```python
from build123d import *

# Parameters (mm, degrees)
BOSS_EXTRUDE1_DEPTH = 222.57
CUT_EXTRUDE2_START  = -10
CUT_EXTRUDE2_DEPTH  = 10
CUT_EXTRUDE3_START  = -10
CUT_EXTRUDE3_DEPTH  = 10


with BuildPart() as part:
    # Sketch1 → Boss-Extrude1 (new body)
    with BuildSketch(Plane.XY):
        with BuildLine():
            Line((0, 150), (0, 130))
            ThreePointArc((0, 130), (-130, 0), (0, -130))
            Line((0, -130), (0, -150))
            ThreePointArc((0, -150), (-150, 0), (0, 150))
        make_face()
    extrude(amount=BOSS_EXTRUDE1_DEPTH)

    # Sketch2 → Cut-Extrude2 (cut)
    with BuildSketch(Plane.XY.offset(222.57).offset(CUT_EXTRUDE2_START)):
        with BuildLine():
            Line((-10, 129.614813968), (-52.842182765, 129.614813968))
            ThreePointArc((-52.842182765, 129.614813968), (-139.972484008, 0), (-52.842182765, -129.614813968))
            Line((-52.842182765, -129.614813968), (-10, -129.614813968))
            ThreePointArc((-10, -129.614813968), (-130, 0), (-10, 129.614813968))
        make_face()
    extrude(amount=-CUT_EXTRUDE2_DEPTH, mode=Mode.SUBTRACT)

    # Sketch3 → Cut-Extrude3 (cut)
    with BuildSketch(Plane(origin=(0, 0, 0), x_dir=(-1, 0, 0), z_dir=(0, 0, -1)).offset(CUT_EXTRUDE3_START)):
        with BuildLine():
            Line((10, 129.614813968), (52.842182765, 129.614813968))
            ThreePointArc((52.842182765, 129.614813968), (139.972484008, 0), (52.842182765, -129.614813968))
            Line((52.842182765, -129.614813968), (10, -129.614813968))
            ThreePointArc((10, -129.614813968), (130, 0), (10, 129.614813968))
        make_face()
    extrude(amount=-CUT_EXTRUDE3_DEPTH, mode=Mode.SUBTRACT)


solid = part.part
```
Input: part model. Units: mm. Frame: model coordinates. A direction names the side the tool comes from. Coordinates: 2 decimals unless noted, no trailing zeros. Write each loop counter-clockwise with the first axis right and the second up, starting at its lowest first coordinate (ties: lowest second). Pieces come first, ordered by that corner, then holes.
1) Section D-D on z = 176.5. Output: boundary loops of the cut face in (x, y), and give its area (3 significant figures).
2) Section A-A on x = -126.5. Output: boundary loops of the cut face in (y, z), and give its area (3 significant figures).
3) Material intervals for line 1 along Z through (x, y) = (-71, 111); line 2 along Y through (x, z) = (-78.5, 27.5); line 3 along Y through (x, z) = (-75.5, 75), sorted ascending.
4) Mould query, pull axis Y, two halves, no side actions, for faces 1 (the flat face through (0, -140, 110)), 2 (the flat face through (-32, -129.615, 208)), 3 (the cylindrical face through (-149.964, -3.298, 109.727)). Classes: pulls with the +Y half, pulls with the -Y half, needs draft (parallel to the pull), parting line crosses it, or undercut.
5) Section C-C on x = -64. Output: boundary loops of the cut face in (y, z).
6) Pin query (flat end, axial travel): pin 1 Ø8 at (x, z) = (-19, 32.5) entering from +Y; pin 2 Ø6 at (x, z) = (-116.5, 113) entering from +Y; pin 3 Ø4 at (y, z) = (-24.5, 149) entering from -X. Return the tip coordinate at first contact, or that it passes through.
7) Section B-B on y = 0. Output: boundary loops of the cut face in (x, z).
8) Set-up query: faces 4 (the flat face through (0, 140, 110)), 5 (the flat face through (-133, 1, 10)). Return all of +Z, -Z, +X, -X, +Y, -Y with unobstructed straight access to the full face (end or side cutting, diameter ignored); none if empty.
Check result:
1. outline: (0, -150) - (0, -130) arc R130 cw to (0, 130) - (0, 150) arc R150 ccw to start
1. area: 8,800 mm2
2. outline: (-80.61, 0) - (-29.96, 0) - (-29.96, 10) - (-59.92, 10) - (-59.92, 20) - (-29.96, 20) - (-29.96, 202.57) - (-59.92, 202.57) - (-59.92, 212.57) - (-29.96, 212.57) - (-29.96, 222.57) - (-80.61, 222.57) - close; (29.96, 0) - (80.61, 0) - (80.61, 222.57) - (29.96, 222.57) - (29.96, 212.57) - (59.92, 212.57) - (59.92, 202.57) - (29.96, 202.57) - (29.96, 20) - (59.92, 20) - (59.92, 10) - (29.96, 10) - close
2. area: 21,300 mm2
3. line 1: z = 0 to 10, 20 to 202.57, 212.57 to 222.57
3. line 2: y = -127.82 to -103.62, 103.62 to 127.82
3. line 3: y = -129.61 to -105.83, 105.83 to 129.61
4. face 1: needs draft
4. face 2: undercut
4. face 3: parting line crosses it
5. outline: (-135.66, 0) - (-113.15, 0) - (-113.15, 10) - (-124.48, 10) - (-124.48, 20) - (-113.15, 20) - (-113.15, 202.57) - (-124.48, 202.57) - (-124.48, 212.57) - (-113.15, 212.57) - (-113.15, 222.57) - (-135.66, 222.57) - close; (113.15, 0) - (135.66, 0) - (135.66, 222.57) - (113.15, 222.57) - (113.15, 212.57) - (124.48, 212.57) - (124.48, 202.57) - (113.15, 202.57) - (113.15, 20) - (124.48, 20) - (124.48, 10) - (113.15, 10) - close
6. pin 1: stops at y = 149.25
6. pin 2: stops at y = 98.07
6. pin 3: stops at x = -148.3
7. outline: (-150, 0) - (-130, 0) - (-130, 10) - (-139.97, 10) - (-139.97, 20) - (-130, 20) - (-130, 202.57) - (-139.97, 202.57) - (-139.97, 212.57) - (-130, 212.57) - (-130, 222.57) - (-150, 222.57) - close
8. face 4: +Z, -Z, +X, +Y, -Y
8. face 5: +X
